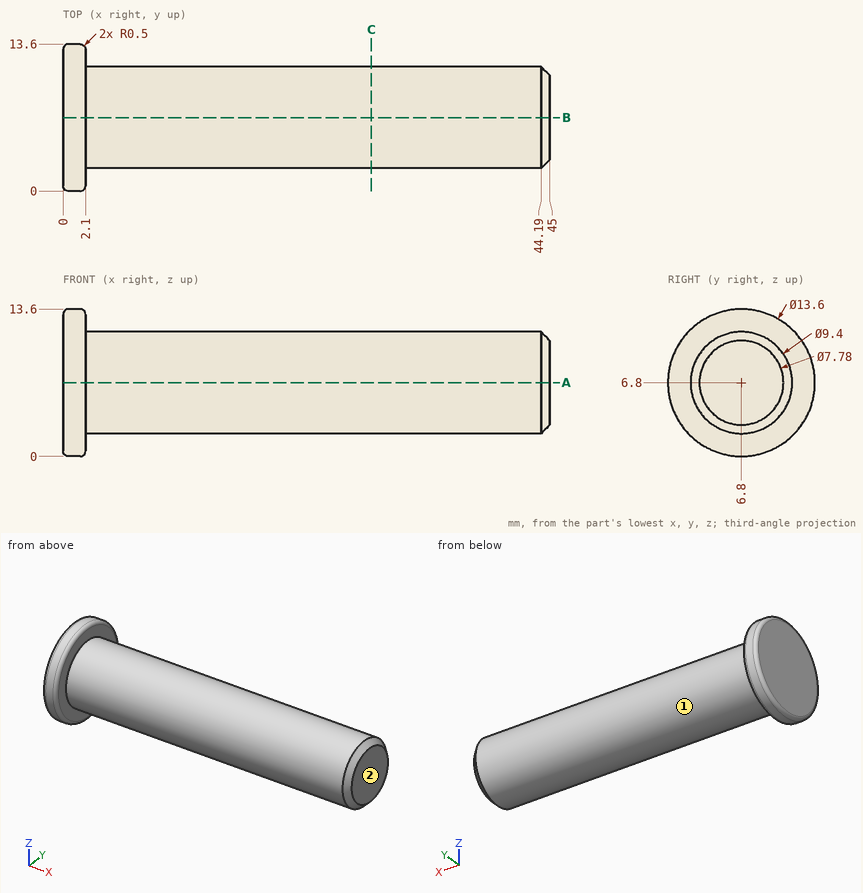
Part print with two shaded views. Sizes in mm from the minimum x, y, z corner. A direction names the side the tool comes from. Give positions to 0.01 mm unless a question says otherwise; leave off trailing zeros. Write each loop counter-clockwise with the first axis right and the second up, starting at its lowest first coordinate (ties: lowest second). Pieces come first, ordered by that corner, then holes.
1) Cut at A-A on z = 6.8. Write the cut outline in (x, y), then the cut area to 3 significant figures.
Resolved:
outline: (0, 0.5) arc R0.5 ccw to (0.5, 0) - (1.6, 0) arc R0.5 ccw to (2.1, 0.5) - (2.1, 2.1) - (44.19, 2.1) - (45, 2.91) - (45, 10.69) - (44.19, 11.5) - (2.1, 11.5) - (2.1, 13.1) arc R0.5 ccw to (1.6, 13.6) - (0.5, 13.6) arc R0.5 ccw to (0, 13.1) - close
area: 431 mm2
2) Which spindle directions (+Z, -Z, +X, -X, +Y, -Y) get a long thin tool onto all of the face, cutting with end or side? Do the marked faces 1 and 2. Say none if no direction does.
Resolved:
face 1: +X
face 2: +Z, -Z, +X, +Y, -Y
3) Cut at C-C on x = 28.5. Write the cut outline in (y, z).
Resolved:
outline: circle Ø9.4 at (6.8, 6.8)
4) Probe L1, parallel to X at y = 4.5, z = 2.5; L2, parallel to Y at x = 22.5, z = 6.75; L3, parallel to Z at x = 27, y = 7.5. List the from-to ranges inside material, lowest first.
Resolved:
L1: x = 0 to 2.1
L2: y = 2.1 to 11.5
L3: z = 2.15 to 11.45
5) Pin check, flat tips, straight feed: pin 1 (6 mm diameter, centred on x = 16, y = 5, fed in from -Z); pin 2 (4 mm diameter, centred on x = 39.5, y = 5, fed in from +Z); pin 3 (1.5 mm diameter, centred on x = 19.5, y = 4.5, fed in from -Z). Stop position of each tip, or through.
Resolved:
pin 1: stops at z = 2.1
pin 2: stops at z = 11.5
pin 3: stops at z = 2.36
